The model under review builds one solid part; all positions refer to its coordinate system, in mm. A direction names the side the tool comes from. Give positions to 0.01 mm unless a question says otherwise; leave off trailing zeros. Order: outer loops, then holes, each group sorted by start corner. A loop starts at its lowest first (then second) coordinate and runs counter-clockwise, first axis right, second up. Notation, with made-up numbers: (57.5, 0.5) - (99.5, 0.5) arc R23 ccw to (99.5, 31.5) - close; hole circle Ø5 at (80, -2.75). An arc over 180 degrees is marked (long way). Use CSV: the item, a comma, the result in double quotes.
```python
from build123d import *

# Parameters (mm, degrees)
SKETCH1_R               = 9.9
SKETCH1_R_2             = 4.1005
BOSS_EXTRUDE1_DEPTH     = 0.889
SKETCH2_R               = 9.9
SKETCH2_W               = 12.9
SKETCH2_H               = 13.2048
BOSS_EXTRUDE2_DEPTH     = 5.4086
SKETCH3_R               = 14.9
SKETCH3_W               = 12.9
SKETCH3_H               = 13.2048
BOSS_EXTRUDE3_DEPTH     = 5
CUT_EXTRUDE6_DEPTH      = 24.909323825
CUT_EXTRUDE6_DEPTH_BACK = 24.909323825
SKETCH4_R               = 1.05
BOSS_EXTRUDE4_START     = 0.5
SKETCH5_R               = 9.9
SKETCH5_R_2             = 4.1005
BOSS_EXTRUDE4_DEPTH     = 0.5
BOSS_EXTRUDE5_START     = 2
SKETCH6_R               = 9.9
SKETCH6_R_2             = 3.587456629
BOSS_EXTRUDE5_DEPTH     = 2
FILLET1_R               = 1
CUT_EXTRUDE7_DEPTH      = 26.187174628
CUT_EXTRUDE7_DEPTH_BACK = 26.187174628
SKETCH7_R               = 1.05


with BuildPart() as part:
    # Sketch1 → Boss-Extrude1 (new body)
    with BuildSketch(Plane.XY):
        Circle(SKETCH1_R)
        Circle(SKETCH1_R_2, mode=Mode.SUBTRACT)
    extrude(amount=-BOSS_EXTRUDE1_DEPTH)

    # Sketch2 → Boss-Extrude2 (add)
    with BuildSketch(Plane(origin=(0, 0, -0.889), x_dir=(-1, 0, 0), z_dir=(0, 0, -1))):
        with Locations(Location((0, 0, 0), (0, 0, 180))):
            Circle(SKETCH2_R)
        Rectangle(SKETCH2_W, SKETCH2_H, mode=Mode.SUBTRACT)
    extrude(amount=BOSS_EXTRUDE2_DEPTH)

    # Sketch3 → Boss-Extrude3 (add)
    with BuildSketch(Plane(origin=(0, 0, -6.2976), x_dir=(-1, 0, 0), z_dir=(0, 0, -1))):
        Circle(SKETCH3_R)
        Rectangle(SKETCH3_W, SKETCH3_H, mode=Mode.SUBTRACT)
    extrude(amount=BOSS_EXTRUDE3_DEPTH)

    # Sketch4 → Cut-Extrude6 (cut, two sides: drawn at the far end of the back side and taken through both)
    with BuildSketch(Plane.XY.offset(-CUT_EXTRUDE6_DEPTH_BACK)):
        with Locations((-7.549511775, 0.085860102)):
            Circle(SKETCH4_R)
        with Locations((7.55, 0)):
            Circle(SKETCH4_R)
    extrude(amount=CUT_EXTRUDE6_DEPTH + CUT_EXTRUDE6_DEPTH_BACK, mode=Mode.SUBTRACT)

    # Sketch5 → Boss-Extrude4 (add)
    with BuildSketch(Plane.XY.offset(BOSS_EXTRUDE4_START)):
        Circle(SKETCH5_R)
        Circle(SKETCH5_R_2, mode=Mode.SUBTRACT)
    extrude(amount=-BOSS_EXTRUDE4_DEPTH)

    # Sketch6 → Boss-Extrude5 (add)
    with BuildSketch(Plane.XY.offset(0.5).offset(BOSS_EXTRUDE5_START)):
        Circle(SKETCH6_R)
        Circle(SKETCH6_R_2, mode=Mode.SUBTRACT)
    extrude(amount=-BOSS_EXTRUDE5_DEPTH)

    # Fillet1
    fillet1_edges = [part.edges().sort_by_distance(p)[0] for p in [
        (14.9, 0, -11.2976),
    ]]
    fillet(fillet1_edges, radius=FILLET1_R)

    # Sketch7 → Cut-Extrude7 (cut, two sides: drawn at the far end of the back side and taken through both)
    with BuildSketch(Plane.XY.offset(2.5).offset(-CUT_EXTRUDE7_DEPTH_BACK)):
        with Locations((7.55, 0)):
            Circle(SKETCH7_R)
        with Locations((-7.549511775, 0.085860102)):
            Circle(SKETCH7_R)
    extrude(amount=CUT_EXTRUDE7_DEPTH + CUT_EXTRUDE7_DEPTH_BACK, mode=Mode.SUBTRACT)


solid = part.part
```
Item 1: Tool access review of faces 5 (the face through (-9, 0, -11.298)), 6 (the face through (0, -6.602, -6)), 7 (the face through (-3, -10, -6.298)): name each direction out of +Z, -Z, +X, -X, +Y, -Y from which nothing blocks a thin tool from reaching the whole face with its end or side.
Results list:
face 5,"-Z, +X, -X, +Y, -Y"
face 6,"-Z"
face 7,"+Z"
Item 2: Mouldability with a two-part tool opening along Y and no side actions: class faces 1 (the face through (6.45, -2, -6)), 2 (the face through (-8.6, 0.1, -4.5)), 3 (the face through (4, 0, 2.5)), 4 (the face through (9.443, 2.974, -1.837)) as pulls with the +Y half, pulls with the -Y half, needs draft (parallel to the pull), parting line crosses it, or undercut.
Results list:
face 1,"undercut"
face 2,"undercut"
face 3,"needs draft"
face 4,"parting line crosses it"
Item 3: Clearance check with flat-ended pins moving along their axes: pin 1 (5 mm diameter, centred on x = 3, z = -7, fed in from +Y); pin 2 (6 mm diameter, centred on y = -4.5, z = -3.5, fed in from -X); pin 3 (3 mm diameter, centred on x = -1, z = -5, fed in from -Y); pin 4 (6.5 mm diameter, centred on x = 0, y = 0, fed in from +Z). State where each tip first meets the part, or that it passes through.
Results list:
pin 1,"stops at y = 14.89"
pin 2,"stops at x = -14.5"
pin 3,"stops at y = -14.9"
pin 4,"passes through"
Item 4: Take a section at A-A, the plane x = 0. Give the boundary of the cut face in (y, z).
Results list:
outline,"(-14.9, -10.3) arc R1 ccw to (-13.9, -11.3) - (-6.6, -11.3) - (-6.6, -0.89) - (-4.1, -0.89) - (-4.1, 0.5) - (-3.59, 0.5) - (-3.59, 2.5) - (-9.9, 2.5) - (-9.9, -6.3) - (-14.9, -6.3) - close; (3.59, 0.5) - (4.1, 0.5) - (4.1, -0.89) - (6.6, -0.89) - (6.6, -11.3) - (13.9, -11.3) arc R1 ccw to (14.9, -10.3) - (14.9, -6.3) - (9.9, -6.3) - (9.9, 2.5) - (3.59, 2.5) - close"
Item 5: Wall thickness on L1, parallel to Y at x = 0, z = 1.3; L2, parallel to Y at x = 0, z = -0.45; L3, parallel to Z at x = -7, y = 9: over which ranges is each line inside the solid? List them lowest first.
Results list:
L1,"y = -9.9 to -3.59, 3.59 to 9.9"
L2,"y = -9.9 to -4.1, 4.1 to 9.9"
L3,"z = -11.3 to -6.3"
Item 6: Take a section at B-B, the plane z = -1.75. Give the boundary of the cut face in (x, y), and give its area (3 significant figures).
Results list:
outline,"circle Ø19.8 at (0, 0); hole circle Ø2.1 at (-7.55, 0.09); hole (-6.45, -6.6) - (6.45, -6.6) - (6.45, 6.6) - (-6.45, 6.6) - close; hole circle Ø2.1 at (7.55, 0)"
area,"131 mm2"
